Autodesk Fusion 360 part; units mm, degrees
sketch "Sketch1" plane through (0, 0, 0) normal (0, 0, 1) x (1, 0, 0) in component "Motor"
  line L0 (32.5, 9.5) -> (-32.5, 9.5)
  line L1 (-32.5, 9.5) -> (-32.5, -9.5)
  line L2 (-32.5, -9.5) -> (32.5, -9.5)
  line L3 (32.5, -9.5) -> (32.5, 9.5)
  line L4 (32.5, 9.5) -> (-32.5, -9.5) construction
  line L5 (-32.5, 9.5) -> (32.5, -9.5) construction
  dimension "d1" = 65
  dimension "d2" = 19
extrude "Extrude1" add sketch "Sketch1" along normal blind 25 in component "Motor"
extrude "Extrude2" cut 1 faces at (-10.8333, -3.1667, 25) along direction (0, 0, -1) blind 3 in component "Motor"
extrude "Extrude3" cut 1 faces at (-32.5, 3.1667, 14.6667) along direction (1, 0, 0) blind 28.3 in component "Motor"
sketch "Sketch2" plane through (-4.2, 0, 0) normal (-1, 0, 0) x (0, -1, 0) in component "Motor"
  line L0 (9.5, 22) -> (-9.5, 22)
  line L1 (-9.5, 22) -> (-9.5, 0)
  line L2 (-9.5, 0) -> (9.5, 0)
  line L3 (9.5, 0) -> (9.5, 22)
  line L4 (-9.5, 22) -> (9.5, 22)
  line L5 (9.5, 22) -> (9.5, 0)
  line L6 (9.5, 0) -> (-9.5, 0)
  line L7 (-9.5, 0) -> (-9.5, 22)
  line L8 (-7, 19) -> (7, 19)
  line L9 (7, 19) -> (7, 2)
  line L10 (7, 2) -> (-7, 2)
  line L11 (-7, 2) -> (-7, 19)
  line L12 (-6, 18) -> (6, 18)
  line L13 (6, 18) -> (6, 3)
  line L14 (6, 3) -> (-6, 3)
  line L15 (-6, 3) -> (-6, 18)
extrude "Extrude4" add sketch "Sketch2" along normal blind 28.3 contours L8 L9 L10 L11 | L12 L13 L14 L15 in component "Motor"
fillet "Fillet1" radius 5 2 edges at (32.5, 0, 22) (32.5, 0, 0) in component "Motor"
extrude "Extrude5" cut 1 faces at (-32.5, 2.3333, 7.6667) along direction (1, 0, 0) blind 14.15 in component "Motor"
extrude "Extrude6" add sketch "Sketch2" along normal blind 28.3 contours L12 L13 L14 L15 in component "Motor"
fillet "Fillet2" radius 2.5 1 faces at (-32.5, 2, 13) in component "Motor"
sketch "Sketch3" plane through (0, -9.5, 0) normal (0, -1, 0) x (1, 0, 0) in component "Motor"
  arc A0 (27.5, 0) -> (32.5, 5) centre (27.5, 5) ccw
  line L0 (32.5, 5) -> (32.5, 17)
  arc A1 (32.5, 17) -> (27.5, 22) centre (27.5, 17) ccw
  line L1 (27.5, 22) -> (-4.2, 22)
  line L2 (-4.2, 22) -> (-4.2, 0)
  line L3 (-4.2, 0) -> (27.5, 0)
  line L4 (-4.2, 22) -> (27.6, 22)
  line L5 (32.6, 17) -> (32.6, 5)
  line L6 (27.6, 0) -> (-4.2, 0)
  line L7 (-4.2, 0) -> (-4.2, 22)
  arc A2 (32.6, 17) -> (27.6, 22) centre (27.6, 17) ccw
  arc A3 (27.6, 0) -> (32.6, 5) centre (27.6, 5) ccw
  circle A4 centre (23, 11) radius 3
  point P0 (32.6, 22)
  dimension "d19" = 36.8
  dimension "d20" = 5
  dimension "d21" = 6
extrude "Extrude7" cut sketch "Sketch3" against normal blind 56 contours A4 in component "Motor"
component "Motor" placed x (1, 0, 0) y (0, 1, 0) z (0, 0, 1) at (0, 0, 0)
equation "d13 = ( -28.3 / 2 ) * 1 mm"
The listing builds one solid part. Answer for the finished solid, in the listing's coordinates (mm). A direction names the side the tool comes from. Round coordinates to 2 decimals unless told otherwise and drop trailing zeros. Order: outer loops, then holes, each group sorted by start corner. A loop starts at its lowest first (then second) coordinate and runs counter-clockwise, first axis right, second up. Notation, with made-up numbers: M 48,49.5 L 84,49.5 A12 cw 84,67.5 Z; hole C 62,47 d11. An arc over 180 degrees is marked long. Answer in a Markdown table with one row per item. Add a question column.
1) The part is cut by section B-B on y = 0.25. Determine the outline of the cut face in (x, z).
2) The part is cut by section C-C on z = 11. Determine the outline of the cut face in (x, y), plus the area to 3 significant figures.
3) The part is cut by section D-D on z = 14.75. Determine the outline of the cut face in (x, y), plus the area to 3 significant figures.
4) The part is cut by section A-A on x = 23. Determine the outline of the cut face in (y, z), plus the area to 3 significant figures.
5) Flat-ended cylindrical pins translate along their axes: pin 1 Ø9.5 at (x, y) = (-23.5, -2.5) entering from -Z; pin 2 Ø1.5 at (x, z) = (-7.5, 9) entering from +Y; pin 3 Ø7 at (x, y) = (-11, 2) entering from +Z. Find the tip coordinate at first contact, or state that the pin passes through.
6) Consider line 1 along Z through (x, y) = (23, -5.5); line 2 along Y through (x, z) = (-7.5, 16.75); line 3 along Z through (x, y) = (-12.5, -4.5). Determine where each line is inside the solid, lowest interval first. Write a range as from..to.
7) Which of the six approach directions +Z, -Z, +X, -X, +Y, -Y give full straight-line access (tool end or side, diameter ignored) to faces 5 (the face through (-24, 0, 18)), 6 (the face through (-24, 6, 10)), 7 (the face through (-24, -6, 11))?
8) Determine the mould class of faces 1 (the face through (31, 0.13, 20.57)), 2 (the face through (20, 0, 11)), 3 (the face through (-11, 7, 10)), 4 (the face through (-32, 5, 11)) for opening direction X: pulls with the +X half, pulls with the -X half, needs draft (parallel to the pull), parting line crosses it, or undercut.
Findings below:
| question | item | result |
|---|---|---|
| 1 | outline | M -32.5,5.5 A2.5 ccw -30,3 L -18.35,3 L -18.35,2 L -4.2,2 L -4.2,0 L 27.5,0 A5 ccw 32.5,5 L 32.5,17 A5 ccw 27.5,22 L -4.2,22 L -4.2,19 L -18.35,19 L -18.35,18 L -30,18 A2.5 ccw -32.5,15.5 Z; hole C 23,11 d6 |
| 2 | outline | M -32.5,-3.5 A2.5 ccw -30,-6 L -18.35,-6 L -18.35,-7 L -4.2,-7 L -4.2,-9.5 L 20,-9.5 L 20,9.5 L -4.2,9.5 L -4.2,7 L -18.35,7 L -18.35,6 L -30,6 A2.5 ccw -32.5,3.5 Z; M 26,-9.5 L 32.5,-9.5 L 32.5,9.5 L 26,9.5 Z |
| 2 | area | 949 mm² |
| 3 | outline | M -32.5,-3.5 A2.5 ccw -30,-6 L -18.35,-6 L -18.35,-7 L -4.2,-7 L -4.2,-9.5 L 32.5,-9.5 L 32.5,9.5 L -4.2,9.5 L -4.2,7 L -18.35,7 L -18.35,6 L -30,6 A2.5 ccw -32.5,3.5 Z |
| 3 | area | 1,060 mm² |
| 4 | outline | M -9.5,0 L 9.5,0 L 9.5,8 L -9.5,8 Z; M -9.5,14 L 9.5,14 L 9.5,22 L -9.5,22 Z |
| 4 | area | 304 mm² |
| 5 | pin 1 | stops at z = 3 |
| 5 | pin 2 | stops at y = 7 |
| 5 | pin 3 | stops at z = 19 |
| 6 | line 1 | z = 0..8, 14..22 |
| 6 | line 2 | y = -7..7 |
| 6 | line 3 | z = 2..19 |
| 7 | face 5 | +Z, -X, +Y, -Y |
| 7 | face 6 | +Z, -Z, -X, +Y |
| 7 | face 7 | +Z, -Z, -X, -Y |
| 8 | face 1 | pulls with the +X half |
| 8 | face 2 | undercut |
| 8 | face 3 | needs draft |
| 8 | face 4 | pulls with the -X half |
